Can you work these out from the model? Positions are in its coordinate system, mm. A direction names the side the tool comes from. Round coordinates to 2 decimals unless told otherwise and drop trailing zeros. Loops run counter-clockwise (first coordinate to the right, second up) from the corner with the lowest first, then second, coordinate; pieces in that order, holes last. Notation, with made-up numbers: (74.5, 16) -> (79.5, 16) arc R22 cw to (79.5, 39) -> close; hole circle Ø10 at (-36, 12). An arc over 180 degrees is marked (long way). Answer as a JSON object with one key per item and string values.
```python
from build123d import *

# Parameters (mm, degrees)
SKETCH1_R      = 16.8
EXTRUDE1_DEPTH = 7.9
SKETCH2_R      = 9.5123
THREAD_DEPTH   = 16
CHAMFER1_SIZE  = 1.2
CHAMFER2_SIZE  = 0.5
RODHOLE_REACH  = 35.7
SKETCH9_R      = 5.6


with BuildPart() as part:
    # Sketch1 → Extrude1 (new body)
    with BuildSketch(Plane.XY):
        Circle(SKETCH1_R)
    extrude(amount=EXTRUDE1_DEPTH)

    # Sketch2 → THREAD (add)
    with BuildSketch(Plane.XY.offset(7.9)):
        Circle(SKETCH2_R)
    extrude(amount=THREAD_DEPTH)

    # Sketch3 → THREAD END (revolve, cut)
    with BuildSketch(Plane(origin=(0, 0, 0), x_dir=(0, 0, -1), z_dir=(1, 0, 0)), mode=Mode.PRIVATE) as thread_end_sk:
        with BuildLine():
            Line((-11.8877, 8.5), (-11.1123, 8.5))
            ThreePointArc((-11.1123, 8.5), (-10.396495805, 8.796495805), (-10.1, 9.5123))
            Line((-10.1, 9.5123), (-12.9, 9.5123))
            ThreePointArc((-12.9, 9.5123), (-12.603504195, 8.796495805), (-11.8877, 8.5))
        make_face()
    revolve(thread_end_sk.sketch.rotate(Axis((0, 0, 23.9), (0, 0, -1)), 180), axis=Axis((0, 0, 23.9), (0, 0, -1)), mode=Mode.SUBTRACT)

    # Chamfer1
    chamfer1_edges = [part.edges().sort_by_distance(p)[0] for p in [
        (-9.5123, 0, 23.9),
    ]]
    chamfer(chamfer1_edges, length=CHAMFER1_SIZE)

    # Chamfer2
    chamfer2_edges = [part.edges().sort_by_distance(p)[0] for p in [
        (-16.8, 0, 7.9),
    ]]
    chamfer(chamfer2_edges, length=CHAMFER2_SIZE)

    # Sketch9 → RodHole (cut, up to next)
    with BuildSketch(Plane.XY.offset(23.9), mode=Mode.PRIVATE) as rodhole_sk1:
        Circle(SKETCH9_R)
    rodhole_tool1 = extrude(rodhole_sk1.sketch, amount=-RODHOLE_REACH, mode=Mode.PRIVATE) & part.part
    add(rodhole_tool1.solids().sort_by_distance((0, 0, 23.9))[0], mode=Mode.SUBTRACT)


solid = part.part
```
Q1. If I drill on L1, parallel to Y at x = 0, z = 15; L2, parallel to Y at x = 0.5, z = 3, over which ranges is the centre line in solid material (lowest first)? Write a range as [from, to].
Determined:
{"L1": "[-9.51, -5.6], [5.6, 9.51]", "L2": "[-16.79, -5.58], [5.58, 16.79]"}
Q2. I want a section at D-D, the plane z = 3.5. Write out the boundary of the cut face in (x, y), then the cut area to 3 significant figures.
Determined:
{"outline": "circle Ø33.6 at (0, 0); hole circle Ø11.2 at (0, 0)", "area": "788 mm²"}
Q3. I want a section at C-C, the plane z = 16.75. Write out the boundary of the cut face in (x, y), then the cut area to 3 significant figures.
Determined:
{"outline": "circle Ø19.02 at (0, 0); hole circle Ø11.2 at (0, 0)", "area": "186 mm²"}
Q4. I'm going to push flat-ended pins straight in: pin 1 (6 mm diameter, centred on y = 7.5, z = 14, fed in from +X); pin 2 (9 mm diameter, centred on x = 0, y = 0, fed in from -Z); pin 3 (6 mm diameter, centred on y = 9.5, z = 2.5, fed in from +X); pin 4 (2 mm diameter, centred on x = 2.5, y = -4.5, fed in from +Z). Where does each tip first touch, or does it pass through?
Determined:
{"pin 1": "x = 8.38", "pin 2": "through", "pin 3": "x = 15.49", "pin 4": "z = 23.9"}
Q5. On a 3-axis mill with a long thin cutter (end or side, diameter ignored), from which of +Z, -Z, +X, -X, +Y, -Y can I reach the whole of each face in a straight line? I mean faces 1 (the cylindrical face through (8.79, -3.64, 8.98)), 2 (the cylindrical face through (-5.595, 0.246, 12.117)). Say none if no direction works.
Determined:
{"face 1": "+Z", "face 2": "+Z, -Z"}
Q6. We'd pull the mould along Z, two halves only. Please class faces 3 (the flat face through (7, -7, 7.9)), 4 (the cylindrical face through (-8.428, 1.107, 11.495)), 5 (the flat face through (7, 0, 0)): pulls with the +Z half, pulls with the -Z half, needs draft (parallel to the pull), parting line crosses it, or undercut.
Determined:
{"face 3": "pulls with the +Z half", "face 4": "undercut", "face 5": "pulls with the -Z half"}
Q7. I want a section at A-A, the plane y = 0. Write out the boundary of the cut face in (x, z).
Determined:
{"outline": "(-16.8, 0) -> (-5.6, 0) -> (-5.6, 23.9) -> (-8.31, 23.9) -> (-9.51, 22.7) -> (-9.51, 12.9) arc R1.01 cw to (-8.5, 11.89) -> (-8.5, 11.11) arc R1.01 cw to (-9.51, 10.1) -> (-9.51, 7.9) -> (-16.3, 7.9) -> (-16.8, 7.4) -> close; (5.6, 0) -> (16.8, 0) -> (16.8, 7.4) -> (16.3, 7.9) -> (9.51, 7.9) -> (9.51, 10.1) arc R1.01 cw to (8.5, 11.11) -> (8.5, 11.89) arc R1.01 cw to (9.51, 12.9) -> (9.51, 22.7) -> (8.31, 23.9) -> (5.6, 23.9) -> close"}
